from build123d import *

# Parameters (mm, degrees)
F1_DEPTH    = 57.15
F2_W        = 6.35
F2_H        = 25.4
F3_DEPTH    = 25.4
F4_T1_DEPTH = 48.9464301965


# Not quite as in the source:
# - a fillet or chamfer that OpenCascade refuses, or shapes differently, is made with other operations: its cross-section is extruded or revolved along the edge and cut away or added


with BuildPart() as f1:
    # F0 (on Front) → F1 (new body)
    with BuildSketch(Plane.XZ):
        Polygon((36.6440817745, 56.0591582008), (30.2940817745, 56.0591582008), (30.2940817745, 30.6591582008), (-35.7496880067, -46.5469327059), (-32.0828693102, -49.6836091906), (36.6440817745, 30.6591582008), align=None)
    extrude(amount=F1_DEPTH)

    # F2 (on face) → F3 (join)
    with BuildSketch(Plane.YZ.offset(36.6440817745)):
        with Locations((-53.975, 43.3591582008)):
            Rectangle(F2_W, F2_H)
    extrude(amount=F3_DEPTH)

    # F4: fillet of radius 10.16 on 1 edges, made by hand

    # F4_s2 → F4_t1 (cut)
    with BuildSketch(Plane.YZ.offset(36.6440817745)):
        with BuildLine():
            ThreePointArc((-57.15, 30.6591582008), (-52.5357730325, 34.3981176165), (-50.8, 40.0777302794))
            Line((-50.8, 40.0777302794), (-50.8, 30.6591582008))
            Line((-50.8, 30.6591582008), (-57.15, 30.6591582008))
        make_face()
    extrude(amount=F4_T1_DEPTH, mode=Mode.SUBTRACT)


solid = f1.part
Can you work these out from the model? Positions are in its coordinate system, mm. A direction names the side the tool comes from. Coordinates: 2 decimals unless noted, no trailing zeros. Loops run counter-clockwise (first coordinate to the right, second up) from the corner with the lowest first, then second, coordinate; pieces in that order, holes last. Notation, with made-up numbers: (44, 2) - (77, 2) arc R32 cw to (77, 40) - close; hole circle Ø7 at (45, -35.5). An arc over 180 degrees is marked (long way). Answer as a JSON object with one key per item and string values. Group by question number.
Item 1: If we section it at B-B (y = -19.5): List the corners of the cut face in (x, z) for me, plus the area to 3 significant figures.
Item 2: For pin 1 (1 mm diameter, centred on y = -33, z = -33, fed in from +X); pin 2 (2 mm diameter, centred on y = -6, z = -2, fed in from -X); pin 3 (1 mm diameter, centred on y = -50.5, z = -4, fed in from -X), each with a flat end and sliding along its axis, tell me the tip position at first contact or that it passes through.
Item 3: If we section it at A-A (z = 41.5): List the corners of the cut face in (x, y) for me.
Item 4: If we section it at C-C (x = 1): List the corners of the cut face in (y, z) for me.
Item 5: On a 3-axis mill with a long thin cutter (end or side, diameter ignored), from which of +Z, -Z, +X, -X, +Y, -Y can I reach the whole of each face in a straight line? I mean faces 1 (the face through (49, -50.8, 48)), 2 (the face through (8, 0, 3)), 3 (the face through (36, -35, 56.059)), 4 (the face through (30.294, -28, 44)), 5 (the face through (49.17, -52.58, 34.33)). Say none if no direction works.
Item 6: If I drill on L1, parallel to X at y = -15, z = 44; L2, parallel to X at y = -38, z = 12; L3, parallel to Z at x = -18, y = -22.5, over which ranges is the centre line in solid material (lowest first)? Write a range as from..to.
Item 7: If we section it at D-D (z = -24.5): List the corners of the cut face in (x, y) for me, plus the area to 3 significant figures.
Returned:
{
 "1": {"outline": "(-35.75, -46.55) - (-32.08, -49.68) - (36.64, 30.66) - (36.64, 56.06) - (30.29, 56.06) - (30.29, 30.66) - close", "area": "662 mm²"},
 "2": {"pin 1": "stops at x = -17.38", "pin 2": "stops at x = 1.5", "pin 3": "stops at x = 0.22"},
 "3": {"outline": "(30.29, -57.15) - (62.04, -57.15) - (62.04, -50.8) - (36.64, -50.8) - (36.64, 0) - (30.29, 0) - close"},
 "4": {"outline": "(-57.15, -11.01) - (0, -11.01) - (0, -3.59) - (-57.15, -3.59) - close"},
 "5": {"face 1": "+Z, -Z, +X, +Y", "face 2": "+Z, -Z, +X, -X, +Y", "face 3": "+Z, +X, -X, +Y, -Y", "face 4": "+Z, -X, +Y, -Y", "face 5": "-Z, +X, +Y"},
 "6": {"L1": "x = 30.29..36.64", "L2": "x = 14.33..20.68", "L3": "z = -33.22..-25.8"},
 "7": {"outline": "(-16.89, -57.15) - (-10.54, -57.15) - (-10.54, 0) - (-16.89, 0) - close", "area": "363 mm²"}
}
